Could you check a few things on this model? Use its own coordinates, in mm. Coordinates: 2 decimals unless noted, no trailing zeros. Loops run counter-clockwise (first coordinate to the right, second up) from the corner with the lowest first, then second, coordinate; pieces in that order, holes last. Notation, with made-up numbers: (73, -1.75) - (105, -1.75) arc R15 ccw to (105, 8.25) - close; hole circle Ø9 at (-1.5, 35). An arc over 180 degrees is marked (long way). Put each result on its own line as item: value. Start each with the question number.
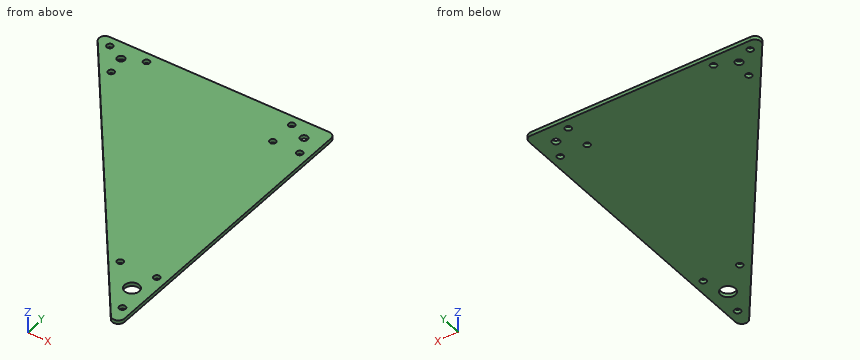
```python
from build123d import *

# Parameters (mm, degrees)
SKETCH_2_R      = 3.1
SKETCH_2_R_2    = 6.05
SKETCH_2_R_3    = 2.55
SKETCH_2_R_4    = 2.6
EXTRUDE_1_DEPTH = 3
FILLET_1_R      = 5


with BuildPart() as part:
    # 草图2 → 凸台-拉伸1 (new body)
    with BuildSketch(Plane.XY):
        Polygon((-180, 15), (15, 15), (15, -245), align=None)
        Circle(SKETCH_2_R, mode=Mode.SUBTRACT)
        with Locations((-150, 0)):
            Circle(SKETCH_2_R, mode=Mode.SUBTRACT)
        with Locations((0, -200)):
            Circle(SKETCH_2_R_2, mode=Mode.SUBTRACT)
        with Locations((-164, 7)):
            Circle(SKETCH_2_R_3, mode=Mode.SUBTRACT)
        with Locations((-134, 7)):
            Circle(SKETCH_2_R_3, mode=Mode.SUBTRACT)
        with Locations((-147.04893552, -15.601419306)):
            Circle(SKETCH_2_R_3, mode=Mode.SUBTRACT)
        with Locations((-15, 7)):
            Circle(SKETCH_2_R_4, mode=Mode.SUBTRACT)
        with Locations((7, -15)):
            Circle(SKETCH_2_R_3, mode=Mode.SUBTRACT)
        with Locations((7, -221)):
            Circle(SKETCH_2_R_4, mode=Mode.SUBTRACT)
        with Locations((-23, -181)):
            Circle(SKETCH_2_R_4, mode=Mode.SUBTRACT)
        with Locations((7, -181)):
            Circle(SKETCH_2_R_4, mode=Mode.SUBTRACT)
        with Locations((-15, -15)):
            Circle(SKETCH_2_R_3, mode=Mode.SUBTRACT)
    extrude(amount=EXTRUDE_1_DEPTH)

    # 圆角1
    fillet_1_edges = [part.edges().sort_by_distance(p)[0] for p in [
        (-180, 15, 1.5),
        (15, 15, 1.5),
        (15, -245, 1.5),
    ]]
    fillet(fillet_1_edges, radius=FILLET_1_R)


solid = part.part
```
(1) I want a section at A-A on y = -200. List the corners of the cut face in (x, z) for me.
(2) I want a section at B-B on x = 0. List the corners of the cut face in (y, z) for me, and give its area (3 significant figures).
(3) I want a section at D-D on y = -9. List the corners of the cut face in (x, z) for me, and give its area (3 significant figures).
(4) I need wall thicknesses on L1, parallel to Y at x = -15, z = 0.75; L2, parallel to X at y = -181, z = 1.9; L3, parallel to Y at x = 7, z = 1.5. Which ranges of each line are inside material? Lowest first, please. Write a range as [from, to].
(5) I want a section at C-C on z = 0.45. Count the separate pieces of the cut face and the enclosed holes in it, and give its area (3 significant figures).
Answer sheet:
1. outline: (-18.75, 0) - (-6.05, 0) - (-6.05, 3) - (-18.75, 3) - close; (6.05, 0) - (15, 0) - (15, 3) - (6.05, 3) - close
2. outline: (-225, 0) - (-206.05, 0) - (-206.05, 3) - (-225, 3) - close; (-193.95, 0) - (-3.1, 0) - (-3.1, 3) - (-193.95, 3) - close; (3.1, 0) - (15, 0) - (15, 3) - (3.1, 3) - close
2. area: 665 mm^2
3. outline: (-162, 0) - (15, 0) - (15, 3) - (-162, 3) - close
3. area: 531 mm^2
4. L1: y = [-205, -17.55], [-12.45, 4.4], [9.6, 15]
4. L2: x = [-33, -25.6], [-20.4, 4.4], [9.6, 15]
4. L3: y = [-234, -223.6], [-218.4, -183.6], [-178.4, -17.55], [-12.45, 15]
5. separate pieces: 1
5. enclosed holes: 12
5. area: 24,900 mm^2
